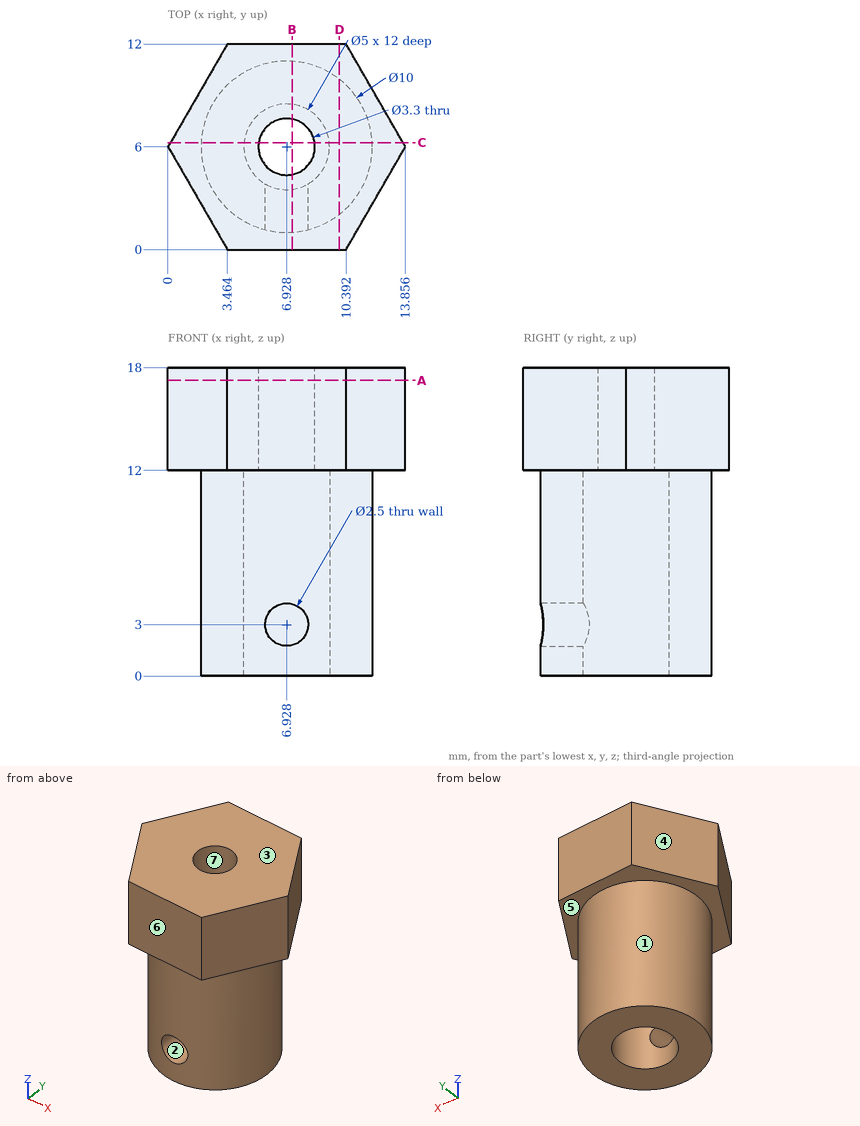
The figure shows three views and two pictorial views of one solid part (mm, origin at its lowest corner). Answer the questions. A direction names the side the tool comes from. Round coordinates to 2 decimals unless told otherwise and drop trailing zeros. Order: outer loops, then holes, each group sorted by start corner. A loop starts at its lowest first (then second) coordinate and runs counter-clockwise, first axis right, second up. Notation, with made-up numbers: (59, 8) - (115, 8) arc R26 ccw to (115, 44) - close; hole circle Ø9 at (14.25, -12.5). An arc over 180 degrees is marked (long way). Write item = value, one per line. Start each with the question number.
1) Section B-B, the plane x = 7.25 is taken. Write down the section's boundary in (y, z), plus the area to 3 significant figures.
2) Section A-A, the plane z = 17.25 is taken. Write down the section's boundary in (x, y).
3) Straight lines are drawn through the part: L1, parallel to Z at x = 4, y = 0.5; L2, parallel to X at y = 1.65, z = 3 (1 decimal); L3, parallel to Y at x = 8.75, z = 3 (1 decimal). For each, find the intervals that lie inside material, in ascending order.
4) Section C-C, the plane y = 6.25 is taken. Write down the section's boundary in (x, z) (1 decimal).
5) Section D-D, the plane x = 10 is taken. Write down the section's boundary in (y, z) (1 decimal), plus the area to 3 significant figures.
6) Given pin 1 (8 mm diameter, centred on x = 4.5, z = 11.5, fed in from +Y); pin 2 (2 mm diameter, centred on x = 6.93, z = 3, fed in from -Y); pin 3 (5 mm diameter, centred on x = 9.5, z = 5, fed in from +Y), each flat-ended and moving along its own axis, determine where each tip first touches the part or whether it passes through.
7) For a pull along Y with two mould halves and no side action, classify the marked faces 4, 5, 6 and 7 as released by +Y, released by -Y, zero draft, split by the parting line, or undercut.
8) For the marked faces 1, 2 and 3, determine the directions among +Z, -Z, +X, -X, +Y, -Y from which every point of the face is accessible in a straight line to the end or side of a thin tool.
Results list:
q1.outline = (0, 12) - (1.01, 12) - (1.01, 4.21) - (3.52, 4.21) - (3.52, 12) - (4.38, 12) - (4.38, 18) - (0, 18) - close; (1.01, 0) - (3.52, 0) - (3.52, 1.79) - (1.01, 1.79) - close; (7.62, 12) - (8.48, 12) - (8.48, 0) - (10.99, 0) - (10.99, 12) - (12, 12) - (12, 18) - (7.62, 18) - close
q1.area = 107 mm^2
q2.outline = (0, 6) - (3.46, 0) - (10.39, 0) - (13.86, 6) - (10.39, 12) - (3.46, 12) - close; hole circle Ø3.3 at (6.93, 6)
q3.L1 = 12 to 18
q3.L2 = 4.5 to 5.7, 8.2 to 9.4
q3.L3 = 1.3 to 4.3, 7.7 to 10.7
q4.outline = (0.1, 12) - (1.9, 12) - (1.9, 0) - (4.4, 0) - (4.4, 12) - (5.3, 12) - (5.3, 18) - (0.1, 18) - close; (8.6, 12) - (9.4, 12) - (9.4, 0) - (11.9, 0) - (11.9, 12) - (13.7, 12) - (13.7, 18) - (8.6, 18) - close
q5.outline = (0, 12) - (2.1, 12) - (2.1, 0) - (9.9, 0) - (9.9, 12) - (12, 12) - (12, 18) - (0, 18) - close
q5.area = 167 mm^2
q6.pin_1 = 12
q6.pin_2 = 8.29
q6.pin_3 = 11
q7.face_4 = released by +Y
q7.face_5 = zero draft
q7.face_6 = released by -Y
q7.face_7 = undercut
q8.face_1 = -Z
q8.face_2 = -Y
q8.face_3 = +Z, +X, -X, +Y, -Y
